Check sheet for the modelled part. Datum: model origin and axes. Units: mm. A direction names the side the tool comes from. Round coordinates to 2 decimals unless told otherwise and drop trailing zeros. Order: outer loops, then holes, each group sorted by start corner. A loop starts at its lowest first (then second) coordinate and runs counter-clockwise, first axis right, second up.
(1) Sectioned sample at C-C, the plane y = 13. Count the separate pieces of the cut face and the enclosed holes in it, and give its area (3 significant figures).
(2) Depth check by flat-ended pin: pin 1 (6 mm diameter, centred on x = -92.52, z = 60.75, fed in from -Y); pin 2 (6 mm diameter, centred on x = -55.02, z = 80.75, fed in from +Y). Enter the tip coordinate at first touch or a pass-through.
(3) Sectioned sample at B-B, the plane z = 69.5. Enter the section's corners in (x, y), and give its area (3 significant figures).
(4) Thickness scan on probe 1 along Z at (x, y) = (-30, 13); probe 2 along X at (y, z) = (18, 81); probe 3 along X at (y, z) = (17, 68.5). Record the ranges inside material, lowest first.
(5) Tool access check on faces 4 (the flat face through (-92, 4, 103)), 5 (the cylindrical face through (-101.665, 0.902, 80.373)). Record the directions out of +Z, -Z, +X, -X, +Y, -Y that give a thin tool (end or side, any length) a straight path to the whole face; none if there is none.
(6) Sectioned sample at A-A, the plane x = -78.5. Enter the section's corners in (y, z) (3 decimals), and give its area (3 significant figures).
(7) Mould release check, pull along Z, two halves, no side actions. Record for faces 1 (the cylindrical face through (-54.4, 0.9, 51.61)), 2 (the cylindrical face through (-17.8, 12.11, 98.62)), 3 (the flat face through (-56, 11, 110.751)): released by +Z, released by -Z, zero draft, split by the parting line, or undercut.
```python
from build123d import *

# Parameters (mm, degrees)
SKETCH1_W                                   = 95
SKETCH1_H                                   = 60
BOSS_EXTRUDE1_DEPTH                         = 20
CBORE_FOR_M4_CHEESE_HEAD_SCREW1_D           = 4.3
CBORE_FOR_M4_CHEESE_HEAD_SCREW1_CBORE_D     = 7.2
CBORE_FOR_M4_CHEESE_HEAD_SCREW1_CBORE_DEPTH = 4
F_5_0MM_DOWEL_HOLE1_D                       = 5
FILLET1_R                                   = 3


with BuildPart() as part:
    # Sketch1 → Boss-Extrude1 (new body)
    with BuildSketch(Plane(origin=(0, 0, 0), x_dir=(1, 0, 0), z_dir=(0, 1, 0))):
        with Locations((-55.020594587, -80.750619844)):
            Rectangle(SKETCH1_W, SKETCH1_H)
    extrude(amount=BOSS_EXTRUDE1_DEPTH)

    # CBORE for M4 Cheese Head Screw1 (through all)
    with Locations(Plane(origin=(0, 0, 0), x_dir=(-1, 0, 0), z_dir=(0, -1, 0))):
        with Locations((17.520594587, -60.750619844), (92.520594587, -60.750619844), (92.520594587, -100.750619844), (17.520594587, -100.750619844)):
            CounterBoreHole(CBORE_FOR_M4_CHEESE_HEAD_SCREW1_D / 2, CBORE_FOR_M4_CHEESE_HEAD_SCREW1_CBORE_D / 2, CBORE_FOR_M4_CHEESE_HEAD_SCREW1_CBORE_DEPTH)

    # Ø5.0mm Dowel Hole1 (through all)
    with Locations(Plane(origin=(0, 0, 0), x_dir=(-1, 0, 0), z_dir=(0, -1, 0))):
        with Locations((30.020594587, -80.750619844), (55.020594587, -80.750619844), (80.020594587, -80.750619844), (55.020594587, -68.250619844), (55.020594587, -93.250619844)):
            Hole(F_5_0MM_DOWEL_HOLE1_D / 2)

    # Fillet1
    fillet1_edges = [part.edges().sort_by_distance(p)[0] for p in [
        (-55.020594587, 0, 50.750619844),
        (-7.520594587, 0, 80.750619844),
        (-55.020594587, 0, 110.750619844),
        (-102.520594587, 0, 80.750619844),
        (-102.520594587, 10, 50.750619844),
        (-7.520594587, 10, 50.750619844),
        (-7.520594587, 10, 110.750619844),
        (-102.520594587, 10, 110.750619844),
    ]]
    fillet(fillet1_edges, radius=FILLET1_R)


solid = part.part
```
Derived:
1. separate pieces: 1
1. enclosed holes: 9
1. area: 5,540 mm2
2. pin 1: stops at y = 4
2. pin 2: stops at y = 20
3. outline: (-102.52, 3) arc R3 ccw to (-99.52, 0) - (-57.19, 0) - (-57.19, 20) - (-102.52, 20) - close; (-52.86, 0) - (-10.52, 0) arc R3 ccw to (-7.52, 3) - (-7.52, 20) - (-52.86, 20) - close
3. area: 1,810 mm2
4. probe 1: z = 50.75 to 78.25, 83.25 to 110.75
4. probe 2: x = -102.52 to -82.51, -77.53 to -57.51, -52.53 to -32.51, -27.53 to -7.52
4. probe 3: x = -102.52 to -57.51, -52.53 to -7.52
5. face 4: -Y
5. face 5: +Z, -Z, -X, -Y
6. outline: (0, 53.751) arc R3 ccw to (3, 50.751) - (20, 50.751) - (20, 78.766) - (0, 78.766) - close; (0, 82.735) - (20, 82.735) - (20, 110.751) - (3, 110.751) arc R3 ccw to (0, 107.751) - close
6. area: 1,120 mm2
7. face 1: released by -Z
7. face 2: undercut
7. face 3: released by +Z
